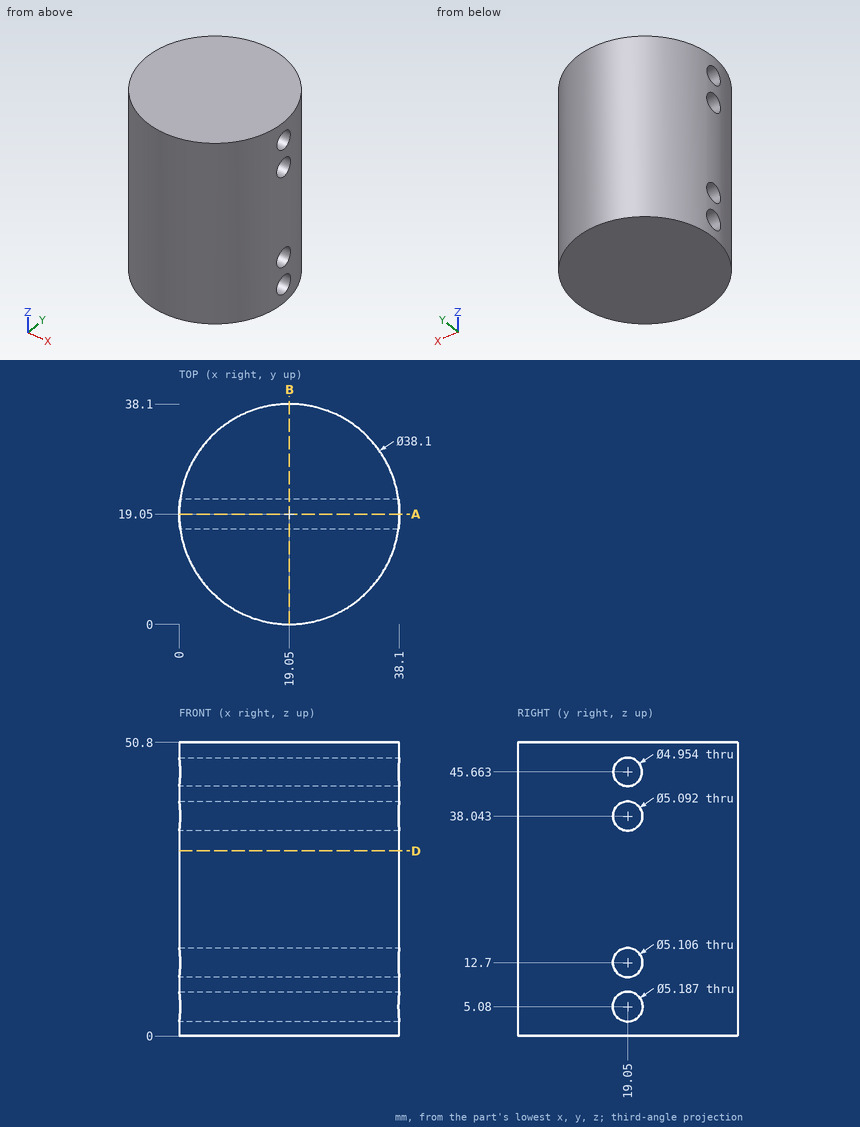
Verification items for this drawing (mm, ordinates from the low corner). Round coordinates to 2 decimals unless told otherwise and drop trailing zeros. Order: outer loops, then holes, each group sorted by start corner. A loop starts at its lowest first (then second) coordinate and runs counter-clockwise, first axis right, second up. Notation, with made-up numbers: (1, 1.25) - (36, 1.25) arc R18 ccw to (36, 7.25) - close; hole circle Ø2 at (38, -17.5). An arc over 180 degrees is marked (long way). Use CSV: the item, a comma, the result in double quotes.
(1) Section check B-B on x = 19.05. State how many separate pieces and enclosed holes the cut face has, and give its area (3 significant figures).
Entries:
separate pieces,"1"
enclosed holes,"4"
area,"1,850 mm^2"
(2) Thickness scan on probe 1 along Y at (x, z) = (25, 5); probe 2 along Y at (x, z) = (15, 12) (1 decimal); probe 3 along Y at (x, z) = (6, 20.5). Record the ranges inside material, lowest first. Write a range as from..to.
Entries:
probe 1,"0.95..16.46, 21.64..37.15"
probe 2,"0.4..16.6, 21.5..37.7"
probe 3,"5.17..32.93"
(3) Section check D-D on z = 32. Record the boundary of the cut face in (x, y), and give its area (3 significant figures).
Entries:
outline,"circle Ø38.1 at (19.05, 19.05)"
area,"1,140 mm^2"
(4) Section check A-A on y = 19.05. Record the boundary of the cut face in (x, z), and give its area (3 significant figures).
Entries:
outline,"(0, 0) - (38.1, 0) - (38.1, 2.49) - (0, 2.49) - close; (0, 7.67) - (38.1, 7.67) - (38.1, 10.15) - (0, 10.15) - close; (0, 15.25) - (38.1, 15.25) - (38.1, 35.5) - (0, 35.5) - close; (0, 40.59) - (38.1, 40.59) - (38.1, 43.19) - (0, 43.19) - close; (0, 48.14) - (38.1, 48.14) - (38.1, 50.8) - (0, 50.8) - close"
area,"1,160 mm^2"
(5) Gauge pin test, flat ends, axial feed: pin 1 Ø1 at (x, z) = (28, 25) entering from -Y; pin 2 Ø8 at (x, z) = (16, 16.5) entering from +Y; pin 3 Ø6.5 at (y, z) = (19.05, 5.08) entering from +X; pin 4 Ø3 at (y, z) = (6, 19) entering from +X. Record the tip position at first contact, or that the pin passes through.
Entries:
pin 1,"y = 1.98"
pin 2,"y = 38.1"
pin 3,"x = 38.1"
pin 4,"x = 34.2"
